Can you work these out from the model? Positions are in its coordinate system, mm. Face numbers are marked on the shaded views. A direction names the side the tool comes from. Coordinates: 2 decimals unless noted, no trailing zeros. Order: outer loops, then holes, each group sorted by start corner. A loop starts at its lowest first (then second) coordinate and runs counter-clockwise, first axis right, second up. Notation, with made-up numbers: (-18, 44.25) - (39, 44.25) arc R27 cw to (39, 67.25) - close; hole circle Ø10 at (-3.75, 11.25). An arc over 180 degrees is marked (long way). Return JSON: item names as keys, results as strings. Group by question number.
1) Imagine slicing it at B-B (x = 20.75). Write out the boundary of the cut face in (y, z).
2) If we mould it in two halves opening along X, with no side actions, what happens to the marked faces 3, 4 and 5? For each: pulls with the +X half, pulls with the -X half, needs draft (parallel to the pull), parting line crosses it, or undercut.
3) If I drill on line 1 along Z through (x, y) = (5.5, -41.5); line 2 along Z through (x, y) = (20.25, -6.5); line 3 along Y through (x, z) = (19, 1.5), over which ranges is the centre line in solid material (lowest first)?
4) Which directions (+Z, -Z, +X, -X, +Y, -Y) give clear straight access to the entire face, cutting with the end or side of a thin tool? Please do the marked faces 1 and 2.
5) Imagine slicing it at C-C (y = 34). Write out the boundary of the cut face in (x, z) (3 decimals).
6) For pin 1 Ø10 at (y, z) = (-15.5, 10) entering from +X (3 decimals); pin 2 Ø6 at (x, y) = (18.5, -41.5) entering from +Z; pin 3 Ø5 at (x, z) = (6.5, 26.5) entering from +Y; pin 4 Ø12.5 at (x, y) = (19, 16) entering from +Z, each with a flat end and sliding along its axis, tell me the tip position at first contact or that it passes through.
7) Imagine slicing it at A-A (z = 21). Write out the boundary of the cut face in (x, y).
```python
from build123d import *

# Parameters (mm, degrees)
F0_W     = 8.89
F0_H     = 114.3
F1_DEPTH = 6.35
F0_W_2   = 2.54
F2_DEPTH = 25.4
F3_W     = 114.3
F3_H     = 3.81
F4_DEPTH = 5.08
F6_DEPTH = 60.96
F7_W     = 11.43
F7_H     = 25.4
F8_DEPTH = 6.35
F9_ANGLE = 270


with BuildPart() as f1:
    # F0 (on Top) → F1 (new body)
    with BuildSketch(Plane.XY):
        with Locations((-1.27, 0)):
            Rectangle(F0_W, F0_H)
    extrude(amount=F1_DEPTH)

    # F0 (on Top) → F2 (join)
    with BuildSketch(Plane.XY):
        with Locations((4.445, 0)):
            Rectangle(F0_W_2, F0_H)
    extrude(amount=F2_DEPTH)

    # F3 (on face) → F4 (join)
    with BuildSketch(Plane(origin=(3.175, 0, 0), x_dir=(0, -1, 0), z_dir=(-1, 0, 0))):
        with Locations((0, 23.495)):
            Rectangle(F3_W, F3_H)
    extrude(amount=F4_DEPTH)

    # F5 (on face) → F6 (join)
    with BuildSketch(Plane(origin=(-5.715, 0, 0), x_dir=(0, -1, 0), z_dir=(-1, 0, 0))):
        with BuildLine():
            ThreePointArc((-28.5731967743, 6.2570092164), (-31.6139310129, 3.2017607338), (-28.5586825303, 0.1610264952))
            Line((-28.5586825303, 0.1610264952), (-28.5731967743, 6.2570092164))
        make_face()
        with BuildLine():
            Line((-28.5731967743, 6.2570092164), (-28.5586825303, 0.1610264952))
            ThreePointArc((-28.5586825303, 0.1610264952), (-26.4081139286, 1.0563236959), (-25.5179396523, 3.2090178558))
            ThreePointArc((-25.5179396523, 3.2090178558), (-26.4132454924, 5.3668435795), (-28.5731967743, 6.2570092164))
        make_face()
        with BuildLine():
            ThreePointArc((28.5915388763, 6.3205178558), (25.4800388763, 3.2090178558), (28.5915388763, 0.0975178558))
            Line((28.5915388763, 0.0975178558), (28.5915388763, 6.3205178558))
        make_face()
        with BuildLine():
            Line((28.5915388763, 6.3205178558), (28.5915388763, 0.0975178558))
            ThreePointArc((28.5915388763, 0.0975178558), (30.791701626, 1.0088551061), (31.7030388763, 3.2090178558))
            ThreePointArc((31.7030388763, 3.2090178558), (30.791701626, 5.4091806055), (28.5915388763, 6.3205178558))
        make_face()
        with BuildLine():
            ThreePointArc((0, 6.2909908401), (-3.0314611237, 3.2430357116), (0, 0.1950805831))
            Line((0, 0.1950805831), (0, 6.2909908401))
        make_face()
        with BuildLine():
            Line((0.0165388763, 6.2910357116), (0.0165388763, 0.1950357116))
            ThreePointArc((0.0165388763, 0.1950357116), (2.1718003454, 1.0877742425), (3.0645388763, 3.2430357116))
            ThreePointArc((3.0645388763, 3.2430357116), (2.1718003454, 5.3982971806), (0.0165388763, 6.2910357116))
        make_face()
    extrude(amount=F6_DEPTH)

    # F7 (on face) → F8 (join)
    with BuildSketch(Plane.XZ.offset(57.15)):
        with Locations((0, 12.7)):
            Rectangle(F7_W, F7_H)
    extrude(amount=-F8_DEPTH)


with BuildPart() as f1_1:
    # F9: moved
    add(f1.part.rotate(Axis((3.175, 0, 0), (0, -1, 0)), F9_ANGLE))


solid = f1_1.part
```
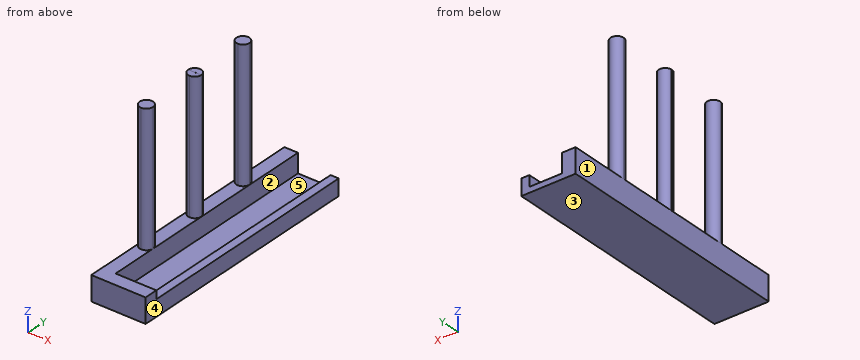
Calculated:
{
 "1": {"outline": "(-57.15, -2.54) - (57.15, -2.54) - (57.15, 0) - (-50.8, 0) - (-50.8, 8.89) - (-57.15, 8.89) - close"},
 "2": {"face 3": "needs draft", "face 4": "pulls with the +X half", "face 5": "undercut"},
 "3": {"line 1": "-2.54 to 8.89", "line 2": "-2.54 to 0", "line 3": "-57.15 to -50.8"},
 "4": {"face 1": "+Z, -Z, -X, +Y, -Y", "face 2": "+Z, +Y"},
 "5": {"outline": "(3.175, -2.54) - (28.575, -2.54) - (28.575, 5.08) - (24.765, 5.08) - (24.765, 0) - (9.525, 0) - (9.525, 8.89) - (3.175, 8.89) - close"},
 "6": {"pin 1": "x = 28.575", "pin 2": "z = 0", "pin 3": "y = 31.61", "pin 4": "z = 5.08"},
 "7": {"outline": "circle Ø6.22 at (6.38, -28.59); circle Ø6.1 at (6.38, 28.57); (3.37, -0.02) arc R3.05 ccw to (9.47, -0.02) - close; (3.37, 0) - (9.47, 0) arc R3.05 ccw to start"}
}
